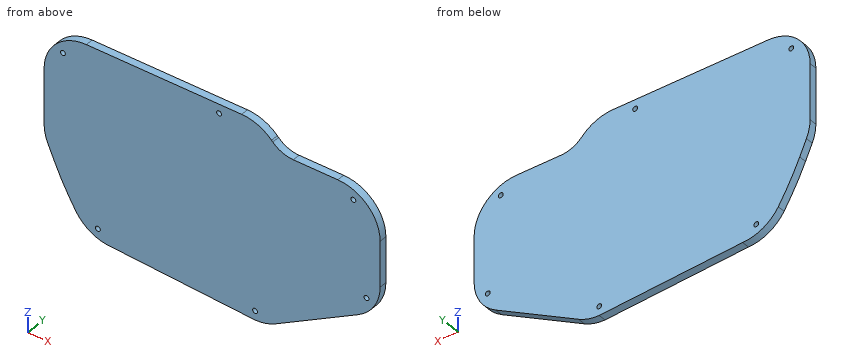
```python
from build123d import *

# Parameters (mm, degrees)
SKETCH2_R           = 1
BOSS_EXTRUDE1_DEPTH = 3.175


with BuildPart() as part:
    # Sketch2 → Boss-Extrude1 (new body)
    with BuildSketch(Plane(origin=(0, 0, 0), x_dir=(1, 0, 0), z_dir=(0, 1, 0))):
        with BuildLine():
            Line((-257.8256366, -105.630010281), (-193.494425739, -105.630010281))
            ThreePointArc((-193.494425739, -105.630010281), (-186.797465673, -104.2979021), (-181.120057068, -100.504378951))
            Line((-181.120057068, -100.504378951), (-180.610104454, -99.994426337))
            ThreePointArc((-180.610104454, -99.994426337), (-176.717024269, -97.393153322), (-172.12482308, -96.479707712))
            Line((-172.12482308, -96.479707712), (-153.649556898, -96.479707712))
            ThreePointArc((-153.649556898, -96.479707712), (-141.275188227, -91.354076382), (-136.149556898, -78.979707712))
            Line((-136.149556898, -78.979707712), (-136.149556898, -60.08207123))
            ThreePointArc((-136.149556898, -60.08207123), (-138.561974219, -51.215569726), (-145.13411106, -44.793605572))
            Line((-145.13411106, -44.793605572), (-179.448460407, -25.681028163))
            ThreePointArc((-179.448460407, -25.681028163), (-183.56493756, -24.031398459), (-187.963906245, -23.469493821))
            Line((-187.963906245, -23.469493821), (-247.380541868, -26.968041449))
            ThreePointArc((-247.380541868, -26.968041449), (-255.809979804, -29.131986673), (-262.154750087, -35.088661324))
            ThreePointArc((-262.154750087, -35.088661324), (-266.895911353, -43.204457303), (-271.025140144, -51.648048015))
            Line((-271.025140144, -51.648048015), (-273.819629856, -57.941117122))
            ThreePointArc((-273.819629856, -57.941117122), (-274.944995262, -61.413292167), (-275.3256366, -65.043382939))
            Line((-275.3256366, -65.043382939), (-275.3256366, -88.130010281))
            ThreePointArc((-275.3256366, -88.130010281), (-270.200005271, -100.504378951), (-257.8256366, -105.630010281))
        make_face()
        with Locations(Location((-147.207602145, -91.127288498, 0), (0, 0, 270))):
            Circle(SKETCH2_R, mode=Mode.SUBTRACT)
        with Locations(Location((-141.795027651, -53.115534334, 0), (0, 0, 270))):
            Circle(SKETCH2_R, mode=Mode.SUBTRACT)
        with Locations(Location((-187.963906245, -27.219493821, 0), (0, 0, 270))):
            Circle(SKETCH2_R, mode=Mode.SUBTRACT)
        with Locations(Location((-253.051529835, -31.941972813, 0), (0, 0, 270))):
            Circle(SKETCH2_R, mode=Mode.SUBTRACT)
        with Locations(Location((-267.548354841, -97.852728522, 0), (0, 0, 270))):
            Circle(SKETCH2_R, mode=Mode.SUBTRACT)
        with Locations(Location((-202.85468144, -101.880010281, 0), (0, 0, 270))):
            Circle(SKETCH2_R, mode=Mode.SUBTRACT)
    extrude(amount=BOSS_EXTRUDE1_DEPTH)


solid = part.part
```
Here's how the part is built. I have some questions about the finished solid (model axes, mm). Coordinates: 2 decimals unless noted, no trailing zeros. Write each loop counter-clockwise with the first axis right and the second up, starting at its lowest first coordinate (ties: lowest second). Pieces come first, ordered by that corner, then holes. Notation, with made-up numbers: M -35,74 L -20,74 A20 cw -20,81 Z; hole C 49.25,6.25 d9. An arc over 180 degrees is marked long. Answer as CSV lines item,"result". Start each with the question number.
Q1. Suppose I cut it at B-B, the plane x = -232. List the corners of the cut face in (y, z) for me (3 decimals), then the cut area to 3 significant figures.
Q2. Suppose I cut it at C-C, the plane x = -264.5. List the corners of the cut face in (y, z) for me (3 decimals), then the cut area to 3 significant figures.
Q3. Will this pin go through, and if not, where does the flat tip stop? pin 1 Ø1.6 at (x, y) = (-163.5, 1.5) entering from +Z.
Q4. Suppose I cut it at A-A, the plane y = 2.4. List the corners of the cut face in (x, z) for me, then the cut area to 3 significant figures.
Q5. I need wall thicknesses on probe 1 along Z at (x, y) = (-162.5, 1.6); probe 2 along X at (y, z) = (1.9, 92); probe 3 along X at (y, z) = (3.05, 31.5). Which ranges of each line are inside material? Lowest first, please. Write a range as [from, to].
Entries:
1,outline,"M 0,26.062 L 3.175,26.062 L 3.175,105.63 L 0,105.63 Z"
1,area,"253 mm²"
2,outline,"M 0,38.931 L 3.175,38.931 L 3.175,104.307 L 0,104.307 Z"
2,area,"208 mm²"
3,pin 1,"stops at z = 96.48"
4,outline,"M -275.33,65.04 A17.5 ccw -273.82,57.94 L -271.03,51.65 A127.26 ccw -262.15,35.09 A17.5 ccw -247.38,26.97 L -187.96,23.47 A17.5 ccw -179.45,25.68 L -145.13,44.79 A17.5 ccw -136.15,60.08 L -136.15,78.98 A17.5 ccw -153.65,96.48 L -172.12,96.48 A12 cw -180.61,99.99 L -181.12,100.5 A17.5 ccw -193.49,105.63 L -257.83,105.63 A17.5 ccw -275.33,88.13 Z; hole C -267.55,97.85 d2; hole C -253.05,31.94 d2; hole C -202.85,101.88 d2; hole C -187.96,27.22 d2; hole C -147.21,91.13 d2; hole C -141.8,53.12 d2"
4,area,"9,720 mm²"
5,probe 1,"z = [35.12, 96.48]"
5,probe 2,"x = [-274.89, -147.7], [-146.72, -141.96]"
5,probe 3,"x = [-259.13, -253.95], [-252.15, -169]"
